```python
from build123d import *

# Parameters (mm, degrees)
EXTRUDE_4_DEPTH = 9


with BuildPart() as part:
    # Эскиз1 → Бобышка-Вытянуть4 (new body)
    with BuildSketch(Plane(origin=(0, 0, 0), x_dir=(0, 0, -1), z_dir=(1, 0, 0))):
        with BuildLine():
            Line((-455, -516.542644104), (-455, 516.556548518))
            Line((-455, 516.556548518), (-248.999999692, 435.905604479))
            add(Edge.make_bspline(
                [(-248.999999692, 435.905604479), (-244.812182794, 427.580683135), (-236.801363167, 410.73826292), (-222.212406758, 376.463926678), (-206.472110198, 332.573595341), (-191.065214882, 278.622516157), (-178.618404528, 223.741954043), (-168.601235151, 168.376182512), (-162.664180548, 121.995794186), (-159.588454358, 84.78039118), (-158.191016915, 56.847307797), (-157.699086883, 28.820440013), (-157.668208508, 0.657149051), (-157.69908686, -27.506141911), (-158.191016904, -55.533009684), (-159.588454431, -83.466093036), (-162.664180797, -120.681496001), (-168.601235656, -167.061884287), (-178.618405136, -222.427655869), (-191.065215126, -277.308218149), (-206.47210996, -331.259297463), (-222.212406313, -375.149628797), (-236.801362845, -409.423964908), (-244.812182664, -426.266385019), (-248.999999692, -434.591306286)],
                knots=[0.002534483, 0.002534483, 0.002534483, 0.002534483, 0.033626078, 0.064717673, 0.126900862, 0.189084052, 0.251267242, 0.313450431, 0.375633621, 0.406725216, 0.43781681, 0.468908405, 0.5, 0.531091595, 0.56218319, 0.593274784, 0.624366379, 0.686549569, 0.748732758, 0.810915948, 0.873099138, 0.935282327, 0.966373922, 0.997465517, 0.997465517, 0.997465517, 0.997465517], degree=3))
            Line((-248.999999692, -434.591306286), (-455, -516.542644104))
        make_face()
        with BuildLine():
            Line((-405, -369.137843077), (-405, -79.83378018))
            ThreePointArc((-405, -79.83378018), (-390.335381972, -44.458495292), (-354.943568764, -29.833812025))
            Line((-354.943568764, -29.833812025), (-260.787453694, -29.940079012))
            ThreePointArc((-260.787453694, -29.940079012), (-223.891969122, -46.256877511), (-211.052398945, -84.501617445))
            add(Edge.make_bspline(
                [(-211.052398945, -84.501617445), (-216.00272922, -138.536584682), (-234.431884839, -238.848455182), (-270.011454394, -336.792856901), (-290.419546493, -382.113233823)],
                knots=[0.6034229, 0.6034229, 0.6034229, 0.6034229, 0.80171145, 0.97615254, 0.97615254, 0.97615254, 0.97615254], degree=3))
            ThreePointArc((-290.419546493, -382.113233823), (-301.450056693, -397.716221108), (-317.52810706, -408.041997779))
            Line((-317.52810706, -408.041997779), (-336.517727965, -415.596487272))
            ThreePointArc((-336.517727965, -415.596487272), (-383.070325953, -410.514851196), (-405, -369.137843077))
        make_face(mode=Mode.SUBTRACT)
        with BuildLine():
            Line((-336.771752099, 416.573644789), (-317.815177046, 409.151966772))
            ThreePointArc((-317.815177046, 409.151966772), (-301.515585195, 398.756977377), (-290.377663678, 382.955736813))
            add(Edge.make_bspline(
                [(-290.377663678, 382.955736813), (-270.15153544, 337.596182562), (-234.790316493, 239.488359394), (-216.31168023, 139.023424648), (-211.259016819, 84.867467904)],
                knots=[0.024188491, 0.024188491, 0.024188491, 0.024188491, 0.1987169, 0.3974338, 0.3974338, 0.3974338, 0.3974338], degree=3))
            ThreePointArc((-211.259016819, 84.867467904), (-224.0817696, 46.549566009), (-261.042812551, 30.222720063))
            Line((-261.042812551, 30.222720063), (-355, 30.222720063))
            ThreePointArc((-355, 30.222720063), (-390.355339059, 44.867381004), (-405, 80.222720063))
            Line((-405, 80.222720063), (-405, 370.014746838))
            ThreePointArc((-405, 370.014746838), (-383.183218455, 411.314942933), (-336.771752099, 416.573644789))
        make_face(mode=Mode.SUBTRACT)
    extrude(amount=EXTRUDE_4_DEPTH)


solid = part.part
```
The listing builds one solid part. Answer for the finished solid, in the listing's coordinates (mm). A direction names the side the tool comes from. Give positions to 0.01 mm unless a question says otherwise; leave off trailing zeros. Write item = value, one per line. Start each with the question number.
1) Which of the six approach directions +Z, -Z, +X, -X, +Y, -Y give full straight-line access (tool end or side, diameter ignored) to faces 1 (the face through (9, 7, 304)), 2 (the face through (4.437, -44.849, 390.722))?
2) Determine the mould class of faces 3 (the face through (4.44, 410.93, 383.74)), 4 (the face through (4.437, 476.796, 353.442)), 5 (the face through (4.437, -474.993, 350.558)) for opening direction Y: +Y half, -Y half, draft (parallel to the pull), parting line (faces both ways), or undercut.
3) Straight lines are drawn through the part: line 1 along Y through (x, z) = (1.5, 345); line 2 along Y through (x, z) = (5.5, 346.5); line 3 along Z through (x, y) = (4.5, -158.5). For each, find the intervals that lie inside material, in ascending order.
4) Each of these flat-tipped pins is pushed along its axis until it touches: pin 1 (4.5 mm diameter, centred on x = 4, z = 306, fed in from +Y); pin 2 (1 mm diameter, centred on x = 5.5, z = 308.5, fed in from +Y); pin 3 (1 mm diameter, centred on x = 5, z = 381, fed in from +Y). Where does it stop, or does it pass through?
5) The part is cut by section A-A, the plane x = 4. Count the separate pieces of the cut face and the enclosed holes in it, and give its area (3 significant figures).
Solutions:
q1.face_1 = +Z, -Z, +X, +Y, -Y
q1.face_2 = +X, -X
q2.face_3 = undercut
q2.face_4 = +Y half
q2.face_5 = -Y half
q3.line_1 = -472.78 to -418.13, -29.85 to 30.22, 419 to 473.49
q3.line_2 = -473.38 to -418.41, -29.84 to 30.22, 419.29 to 474.08
q3.line_3 = 167.8 to 220.94, 405 to 455
q4.pin_1 = 459.1
q4.pin_2 = 459.4
q4.pin_3 = 487.78
q5.separate_pieces = 1
q5.enclosed_holes = 2
q5.area = 129,000 mm²
